from build123d import *

# Parameters (mm, degrees)
F0_W     = 355.6
F0_H     = 355.6
F1_DEPTH = 383.54
F2_T     = -2.54
F4_DEPTH = 25.4


with BuildPart() as f1:
    # F0 (on Top) → F1 (new body)
    with BuildSketch(Plane.XY):
        Rectangle(F0_W, F0_H)
    extrude(amount=F1_DEPTH)

    # F2
    f2_openings = [f1.faces().sort_by_distance(p)[0] for p in [
        (0, 0, 383.54),
    ]]
    offset(amount=F2_T, openings=f2_openings)

    # F3 (on face) → F4 (cut)
    with BuildSketch(Plane.XZ.offset(177.8)):
        Polygon((139.7, 383.54), (-139.7, 383.54), (-63.5, 104.14), (63.5, 104.14), align=None)
    extrude(amount=-F4_DEPTH, mode=Mode.SUBTRACT)


solid = f1.part
The listing builds one solid part. Answer for the finished solid, in the listing's coordinates (mm). A direction names the side the tool comes from. Coordinates: 2 decimals unless noted, no trailing zeros. Write each loop counter-clockwise with the first axis right and the second up, starting at its lowest first coordinate (ties: lowest second). Pieces come first, ordered by that corner, then holes. Notation, with made-up numbers: M 61,83.25 L 85,83.25 A12 cw 85,99.25 Z; hole C -40,-32.75 d9. An arc over 180 degrees is marked long. Write each question's results on one line, items separated by ' | '.
Item 1: The part is cut by section B-B on y = 98. Determine the outline of the cut face in (x, z), and give its area (3 significant figures).
Answer below:
outline: M -177.8,0 L 177.8,0 L 177.8,383.54 L 175.26,383.54 L 175.26,2.54 L -175.26,2.54 L -175.26,383.54 L -177.8,383.54 Z | area: 2,840 mm2
Item 2: Which of the six approach directions +Z, -Z, +X, -X, +Y, -Y give full straight-line access (tool end or side, diameter ignored) to faces 4 (the face through (177.8, -2, 189)), 5 (the face through (101.067, -176.548, 241.884)), 6 (the face through (-175.26, -2, 190))?
Answer below:
face 4: +Z, -Z, +X, +Y, -Y | face 5: +Z, -Y | face 6: +Z
Item 3: The part is cut by section A-A on z = 88.5. Determine the outline of the cut face in (x, y).
Answer below:
outline: M -177.8,-177.8 L 177.8,-177.8 L 177.8,177.8 L -177.8,177.8 Z; hole M -175.26,-175.26 L 175.26,-175.26 L 175.26,175.26 L -175.26,175.26 Z
Item 4: For a pull along Y with two mould halves and no side action, classify faces 1 (the face through (-2, -175.26, 63)), 2 (the face through (-2.5, -177.8, 103.9)), 3 (the face through (-102.133, -176.548, 245.796)) as released by +Y, released by -Y, zero draft, split by the parting line, or undercut.
Answer below:
face 1: undercut | face 2: released by -Y | face 3: zero draft
Item 5: The part is cut by section C-C on x = -55.5. Determine the outline of the cut face in (y, z).
Answer below:
outline: M -177.8,0 L 177.8,0 L 177.8,383.54 L 175.26,383.54 L 175.26,2.54 L -175.26,2.54 L -175.26,104.14 L -177.8,104.14 Z
Item 6: Given P1, Ø2, axis at x = 15, y = -177, coming from the +Z side; P2, Ø10, axis at x = 7, z = 238, coming from the -Y side; P3, Ø6, axis at x = 139.5, y = -49, coming from the +Z side, each flat-ended and moving along its own axis, determine where each tip first touches the part or whether it passes through.
Answer below:
P1: z = 104.14 | P2: y = 175.26 | P3: z = 2.54
Item 7: Consider probe 1 along X at (y, z) = (50, 186); probe 2 along Z at (x, y) = (-62, 1.5). Determine where each line is inside the solid, lowest interval first. Write a range as [from, to].
Answer below:
probe 1: [-177.8, -175.26], [175.26, 177.8] | probe 2: [0, 2.54]
Item 8: The part is cut by section D-D on z = 325.5. Determine the outline of the cut face in (x, y), and give its area (3 significant figures).
Answer below:
outline: M -177.8,-177.8 L -123.87,-177.8 L -123.87,-175.26 L -175.26,-175.26 L -175.26,175.26 L 175.26,175.26 L 175.26,-175.26 L 123.87,-175.26 L 123.87,-177.8 L 177.8,-177.8 L 177.8,177.8 L -177.8,177.8 Z | area: 2,960 mm2
